The model under review builds one solid part; all positions refer to its coordinate system, in mm. A direction names the side the tool comes from. Give positions to 0.01 mm unless a question says otherwise; leave off trailing zeros. Order: outer loops, then holes, each group sorted by start corner. A loop starts at its lowest first (then second) coordinate and runs counter-clockwise, first axis right, second up. Notation, with made-up numbers: (31, -1.5) - (82, -1.5) arc R37 cw to (82, 34.5) - close; hole circle Ø10 at (-12.75, -2). An arc over 180 degrees is marked (long way). Write item = value, one per line. Start each with the question number.
1. We need section A-A, the plane x = 172. Give the boundary of the cut face in (y, z).
2. Wall thickness on probe 1 along X at (y, z) = (-82, 2.2); probe 2 along Y at (x, z) = (156.5, 0.55); probe 3 along Y at (x, z) = (137.5, 1.2): over which ranges is each line inside the solid? List them lowest first.
3. Machinability: for faces 1 (the cylindrical face through (171.48, -108.95, 1.52)), 2 (the flat face through (137, -92.97, 1)), 3 (the flat face through (180, -87.857, 1)), 4 (the flat face through (146, -124.092, 1)), which of the approach directions +Z, -Z, +X, -X, +Y, -Y give a long, thin tool a straight path to every point of the face, cutting with its end or side? Answer none if there is none.
4. We need section B-B, the plane y = -135. Give the boundary of the cut face in (x, z).
5. We need section C-C, the plane z = 0.7. State how many separate pieces and enclosed holes the cut face has, and give its area (3 significant figures).
6. Mouldability with a two-part tool opening along X and no side actions: class faces 5 (the flat face through (132, -106.592, 1)), 6 (the flat face through (127.204, -111, 1)), 7 (the flat face through (177, -115.092, 1)) as pulls with the +X half, pulls with the -X half, needs draft (parallel to the pull), parting line crosses it, or undercut.
7. For P1, Ø1.5, axis at x = 132, z = 1, coming from the -Y side; P2, Ø1.5, axis at x = 142, z = 0.5, coming from the +Y side; P3, Ø0.9, axis at y = -111.5, z = 1, coming from the +X side, all flat-tipped, find the tip position at first contact; note any pin that passes through.
from build123d import *

# Parameters (mm, degrees)
SKETCH1_R           = 1.737885662
SKETCH1_R_2         = 1.873200063
SKETCH1_R_3         = 1.690089146
SKETCH1_R_4         = 1.754205974
SKETCH1_R_5         = 1.7
SKETCH1_R_6         = 4.5
SKETCH1_R_7         = 1.87
SKETCH1_R_8         = 9.5
SKETCH1_W           = 3
SKETCH1_H           = 10
SKETCH1_W_2         = 10
SKETCH1_H_2         = 3
BOSS_EXTRUDE1_DEPTH = 3
FILLET1_R           = 10
FILLET2_R           = 3


with BuildPart() as part:
    # Sketch1 → Boss-Extrude1 (new body)
    with BuildSketch(Plane.XY):
        Polygon((147.061964125, -92.970138098), (147.061964125, -71.856515964), (147.061964125, -67.856515964), (175.843347401, -67.856515964), (175.843347401, -87.856515964), (183.843347401, -87.856515964), (183.843347401, -108.090292187), (170.582125914, -108.090292187), (170.582125914, -115.091712302), (183.843347401, -115.091712302), (183.843347401, -135.887076434), (175.843347401, -135.887076434), (175.843347401, -155.887076434), (147.061964125, -155.887076434), (147.061964125, -151.887076434), (147.061964125, -130.215533927), (127.203791419, -130.215533927), (127.203791419, -111.591712302), (127.203791419, -92.970138098), align=None)
        with Locations((130.520049527, -96.082032258)):
            Circle(SKETCH1_R, mode=Mode.SUBTRACT)
        with Locations((161.520049527, -96.082032258)):
            Circle(SKETCH1_R_2, mode=Mode.SUBTRACT)
        with Locations((130.520049527, -127.114221831)):
            Circle(SKETCH1_R_3, mode=Mode.SUBTRACT)
        with Locations((161.520049527, -127.082032258)):
            Circle(SKETCH1_R_4, mode=Mode.SUBTRACT)
        with Locations((154.157584865, -111.662272701)):
            Circle(SKETCH1_R_5, mode=Mode.SUBTRACT)
        with Locations((145.89014032, -119.788596448)):
            Circle(SKETCH1_R_5, mode=Mode.SUBTRACT)
        with Locations((137.763816574, -111.521151903)):
            Circle(SKETCH1_R_5, mode=Mode.SUBTRACT)
        with Locations((146.031261118, -103.394828157)):
            Circle(SKETCH1_R_5, mode=Mode.SUBTRACT)
        with Locations((145.960700719, -111.591712302)):
            Circle(SKETCH1_R_6, mode=Mode.SUBTRACT)
        with Locations((175.843347401, -96.114221831)):
            Circle(SKETCH1_R_7, mode=Mode.SUBTRACT)
        with Locations((157.960700719, -81.591712302)):
            Circle(SKETCH1_R_8, mode=Mode.SUBTRACT)
        with Locations((157.960700719, -141.591712302)):
            Circle(SKETCH1_R_8, mode=Mode.SUBTRACT)
        with Locations((175.843347401, -127.114221831)):
            Circle(SKETCH1_R_7, mode=Mode.SUBTRACT)
        with Locations((131.960700719, -111.591712302)):
            Rectangle(SKETCH1_W, SKETCH1_H, mode=Mode.SUBTRACT)
        with Locations((145.960700719, -97.591712302)):
            Rectangle(SKETCH1_W_2, SKETCH1_H_2, mode=Mode.SUBTRACT)
        with Locations((145.960700719, -125.591712302)):
            Rectangle(SKETCH1_W_2, SKETCH1_H_2, mode=Mode.SUBTRACT)
        with Locations((166.293610901, -111.591712302)):
            Rectangle(SKETCH1_W, SKETCH1_H, mode=Mode.SUBTRACT)
    extrude(amount=BOSS_EXTRUDE1_DEPTH)

    # Fillet1
    fillet1_edges = [part.edges().sort_by_distance(p)[0] for p in [
        (147.061964125, -67.856515964, 1.5),
        (175.843347401, -67.856515964, 1.5),
        (175.843347401, -155.887076434, 1.5),
        (147.061964125, -155.887076434, 1.5),
    ]]
    fillet(fillet1_edges, radius=FILLET1_R)

    # Fillet2
    fillet2_edges = [part.edges().sort_by_distance(p)[0] for p in [
        (175.843347401, -87.856515964, 1.5),
        (183.843347401, -87.856515964, 1.5),
        (183.843347401, -108.090292187, 1.5),
        (170.582125914, -108.090292187, 1.5),
        (170.582125914, -115.091712302, 1.5),
        (183.843347401, -115.091712302, 1.5),
        (183.843347401, -135.887076434, 1.5),
        (175.843347401, -135.887076434, 1.5),
        (147.061964125, -130.215533927, 1.5),
        (127.203791419, -130.215533927, 1.5),
        (127.203791419, -92.970138098, 1.5),
        (147.061964125, -92.970138098, 1.5),
    ]]
    fillet(fillet2_edges, radius=FILLET2_R)


solid = part.part
Model answer:
q1.outline = (-153.77, 0) - (-114.64, 0) - (-114.64, 3) - (-153.77, 3) - close; (-108.54, 0) - (-69.98, 0) - (-69.98, 3) - (-108.54, 3) - close
q2.probe_1 = 147.06 to 148.47, 167.45 to 175.84
q2.probe_2 = -155.87 to -150.98, -132.2 to -90.98, -72.2 to -67.87
q2.probe_3 = -130.22 to -113.2, -109.84 to -92.97
q3.face_1 = +Z, -Z, +X
q3.face_2 = +Z, -Z, -X, +Y
q3.face_3 = +Z, -Z, +X, +Y
q3.face_4 = +Z, -Z
q4.outline = (147.06, 0) - (151.12, 0) - (151.12, 3) - (147.06, 3) - close; (164.8, 0) - (182.97, 0) - (182.97, 3) - (164.8, 3) - close
q5.separate_pieces = 1
q5.enclosed_holes = 17
q5.area = 2,630 mm2
q6.face_5 = undercut
q6.face_6 = pulls with the -X half
q6.face_7 = needs draft
q7.P1 = -130.22
q7.P2 = -92.97
q7.P3 = 170.58
